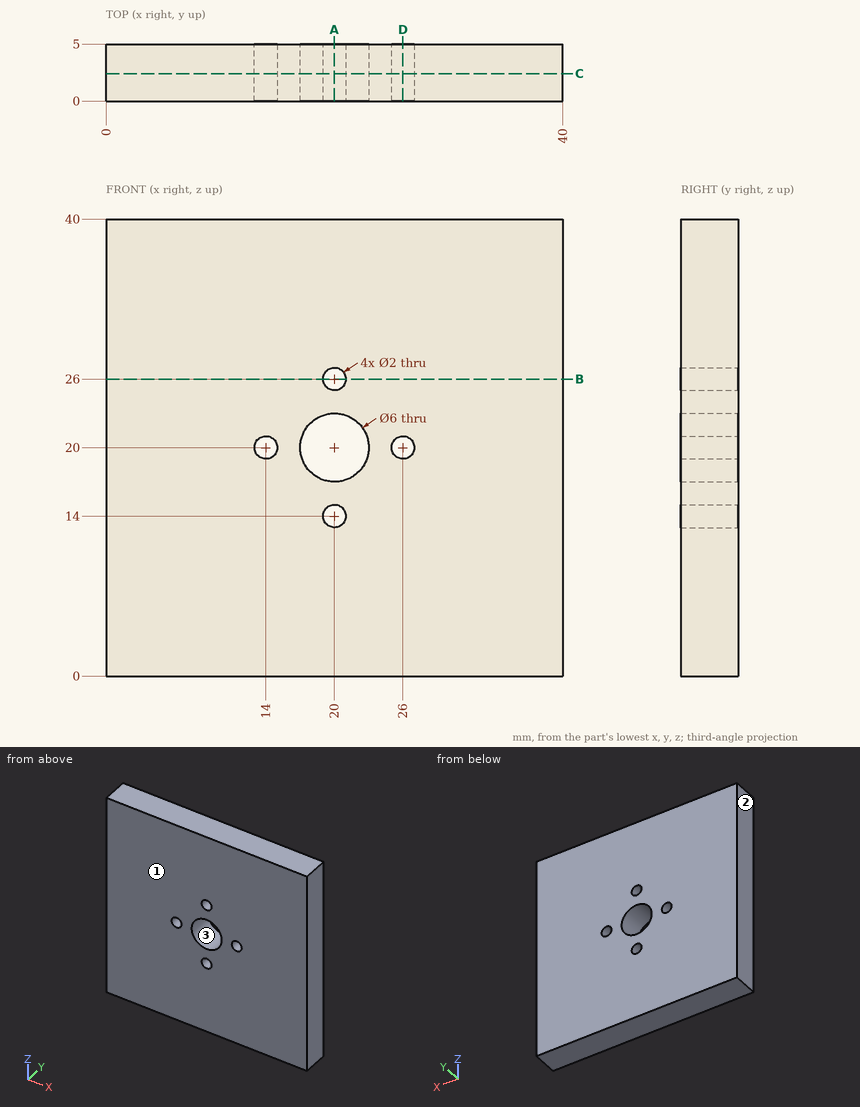
For this review, use the dimensioned drawing (mm, ordinates from the lowest corner) and the shaded views. Round coordinates to 2 decimals unless told otherwise and drop trailing zeros. Write each loop counter-clockwise with the first axis right and the second up, starting at its lowest first coordinate (ties: lowest second). Pieces come first, ordered by that corner, then holes. Notation, with made-up numbers: (41.25, 34) -> (95.25, 34) arc R28 ccw to (95.25, 73) -> close; hole circle Ø7 at (-20.5, -18). An arc over 180 degrees is marked (long way). One line per item, written item: value. Start each with the question number.
Q1. Add section C-C (y = 2.4). Give the boundary of the cut face in (x, z).
Q2. To check wall thickness, follow probe 1 along Z at (x, y) = (20, 3.95); probe 2 along X at (y, z) = (2.3, 26). State the ranges of each line that lie inside material, in increasing order.
Q3. The part is to be moulded in two halves that separate along X. For the marked faces 1, 2 and 3, say which applies: pulls with the +X half, pulls with the -X half, needs draft (parallel to the pull), parting line crosses it, or undercut.
Q4. Add section A-A (x = 20). Give the boundary of the cut face in (y, z).
Q5. Add section D-D (x = 26). Give the boundary of the cut face in (y, z), then the cut area to 3 significant figures.
Q6. Add section B-B (z = 26). Give the boundary of the cut face in (x, y).
Q7. Insertion check: P1, Ø5, axis at x = 20, z = 20, coming from the +Y side. The pin has a flat end and moves straight along its axis. Give the tip position at first contact, or say it passes through.
Response:
1. outline: (0, 0) -> (40, 0) -> (40, 40) -> (0, 40) -> close; hole circle Ø2 at (14, 20); hole circle Ø6 at (20, 20); hole circle Ø2 at (20, 14); hole circle Ø2 at (20, 26); hole circle Ø2 at (26, 20)
2. probe 1: z = 0 to 13, 15 to 17, 23 to 25, 27 to 40
2. probe 2: x = 0 to 19, 21 to 40
3. face 1: needs draft
3. face 2: pulls with the -X half
3. face 3: undercut
4. outline: (0, 0) -> (5, 0) -> (5, 13) -> (0, 13) -> close; (0, 15) -> (5, 15) -> (5, 17) -> (0, 17) -> close; (0, 23) -> (5, 23) -> (5, 25) -> (0, 25) -> close; (0, 27) -> (5, 27) -> (5, 40) -> (0, 40) -> close
5. outline: (0, 0) -> (5, 0) -> (5, 19) -> (0, 19) -> close; (0, 21) -> (5, 21) -> (5, 40) -> (0, 40) -> close
5. area: 190 mm^2
6. outline: (0, 0) -> (19, 0) -> (19, 5) -> (0, 5) -> close; (21, 0) -> (40, 0) -> (40, 5) -> (21, 5) -> close
7. P1: passes through
